from build123d import *

# Parameters (mm, degrees)
F1_DEPTH = 3.175
F2_DEPTH = 4.7498
F3_T     = -1.6002


with BuildPart() as f1:
    # F0 (on Top) → F1 (new body)
    with BuildSketch(Plane.XY):
        with BuildLine():
            Line((-6.9955831819, 8.5962191019), (-38.8090831819, 8.5962191019))
            Line((-38.8090831819, 8.5962191019), (-38.8090831819, 4.6274691019))
            Line((-38.8090831819, 4.6274691019), (-37.2342831819, 4.6274691019))
            ThreePointArc((-37.2342831819, 4.6274691019), (-34.8466831819, 7.0150691019), (-32.4590831819, 4.6274691019))
            Line((-32.4590831819, 4.6274691019), (-29.2840831819, 4.6274691019))
            ThreePointArc((-29.2840831819, 4.6274691019), (-26.8964831819, 7.0150691019), (-24.5088831819, 4.6274691019))
            Line((-24.5088831819, 4.6274691019), (-21.3338831819, 4.6274691019))
            ThreePointArc((-21.3338831819, 4.6274691019), (-18.9462831819, 7.0150691019), (-16.5586831819, 4.6274691019))
            Line((-16.5586831819, 4.6274691019), (-13.3836831819, 4.6274691019))
            ThreePointArc((-13.3836831819, 4.6274691019), (-10.9960831819, 7.0150691019), (-8.6084831819, 4.6274691019))
            Line((-8.6084831819, 4.6274691019), (-6.9955831819, 4.6274691019))
            Line((-6.9955831819, 4.6274691019), (-6.9955831819, 8.5962191019))
        make_face()
        with BuildLine():
            Line((-37.2342831819, 4.6274691019), (-38.8090831819, 4.6274691019))
            Line((-38.8090831819, 4.6274691019), (-38.8090831819, 0.6587191019))
            Line((-38.8090831819, 0.6587191019), (-6.9955831819, 0.6587191019))
            Line((-6.9955831819, 0.6587191019), (-6.9955831819, 4.6274691019))
            Line((-6.9955831819, 4.6274691019), (-8.6084831819, 4.6274691019))
            ThreePointArc((-8.6084831819, 4.6274691019), (-10.9960831819, 2.2398691019), (-13.3836831819, 4.6274691019))
            Line((-13.3836831819, 4.6274691019), (-16.5586831819, 4.6274691019))
            ThreePointArc((-16.5586831819, 4.6274691019), (-18.9462831819, 2.2398691019), (-21.3338831819, 4.6274691019))
            Line((-21.3338831819, 4.6274691019), (-24.5088831819, 4.6274691019))
            ThreePointArc((-24.5088831819, 4.6274691019), (-26.8964831819, 2.2398691019), (-29.2840831819, 4.6274691019))
            Line((-29.2840831819, 4.6274691019), (-32.4590831819, 4.6274691019))
            ThreePointArc((-32.4590831819, 4.6274691019), (-34.8466831819, 2.2398691019), (-37.2342831819, 4.6274691019))
        make_face()
        with BuildLine():
            Line((-37.2342831819, -3.3100308981), (-38.8090831819, -3.3100308981))
            Line((-38.8090831819, -3.3100308981), (-38.8090831819, -7.2787808981))
            Line((-38.8090831819, -7.2787808981), (-6.9955831819, -7.2787808981))
            Line((-6.9955831819, -7.2787808981), (-6.9955831819, -3.3100308981))
            Line((-6.9955831819, -3.3100308981), (-8.6084831819, -3.3100308981))
            ThreePointArc((-8.6084831819, -3.3100308981), (-10.9960831819, -5.6976308981), (-13.3836831819, -3.3100308981))
            Line((-13.3836831819, -3.3100308981), (-16.5586831819, -3.3100308981))
            ThreePointArc((-16.5586831819, -3.3100308981), (-18.9462831819, -5.6976308981), (-21.3338831819, -3.3100308981))
            Line((-21.3338831819, -3.3100308981), (-24.5088831819, -3.3100308981))
            ThreePointArc((-24.5088831819, -3.3100308981), (-26.8964831819, -5.6976308981), (-29.2840831819, -3.3100308981))
            Line((-29.2840831819, -3.3100308981), (-32.4590831819, -3.3100308981))
            ThreePointArc((-32.4590831819, -3.3100308981), (-34.8466831819, -5.6976308981), (-37.2342831819, -3.3100308981))
        make_face()
        with BuildLine():
            Line((-6.9955831819, 0.6587191019), (-38.8090831819, 0.6587191019))
            Line((-38.8090831819, 0.6587191019), (-38.8090831819, -3.3100308981))
            Line((-38.8090831819, -3.3100308981), (-37.2342831819, -3.3100308981))
            ThreePointArc((-37.2342831819, -3.3100308981), (-34.8466831819, -0.9224308981), (-32.4590831819, -3.3100308981))
            Line((-32.4590831819, -3.3100308981), (-29.2840831819, -3.3100308981))
            ThreePointArc((-29.2840831819, -3.3100308981), (-26.8964831819, -0.9224308981), (-24.5088831819, -3.3100308981))
            Line((-24.5088831819, -3.3100308981), (-21.3338831819, -3.3100308981))
            ThreePointArc((-21.3338831819, -3.3100308981), (-18.9462831819, -0.9224308981), (-16.5586831819, -3.3100308981))
            Line((-16.5586831819, -3.3100308981), (-13.3836831819, -3.3100308981))
            ThreePointArc((-13.3836831819, -3.3100308981), (-10.9960831819, -0.9224308981), (-8.6084831819, -3.3100308981))
            Line((-8.6084831819, -3.3100308981), (-6.9955831819, -3.3100308981))
            Line((-6.9955831819, -3.3100308981), (-6.9955831819, 0.6587191019))
        make_face()
    extrude(amount=F1_DEPTH)

    # F0 (on Top) → F2 (join)
    with BuildSketch(Plane.XY):
        with BuildLine():
            Line((-32.4590831819, 4.6274691019), (-37.2342831819, 4.6274691019))
            ThreePointArc((-37.2342831819, 4.6274691019), (-34.8466831819, 2.2398691019), (-32.4590831819, 4.6274691019))
        make_face()
        with BuildLine():
            ThreePointArc((-32.4590831819, 4.6274691019), (-34.8466831819, 7.0150691019), (-37.2342831819, 4.6274691019))
            Line((-37.2342831819, 4.6274691019), (-32.4590831819, 4.6274691019))
        make_face()
        with BuildLine():
            ThreePointArc((-32.4590831819, -3.3100308981), (-34.8466831819, -0.9224308981), (-37.2342831819, -3.3100308981))
            Line((-37.2342831819, -3.3100308981), (-32.4590831819, -3.3100308981))
        make_face()
        with BuildLine():
            Line((-32.4590831819, -3.3100308981), (-37.2342831819, -3.3100308981))
            ThreePointArc((-37.2342831819, -3.3100308981), (-34.8466831819, -5.6976308981), (-32.4590831819, -3.3100308981))
        make_face()
        with BuildLine():
            Line((-24.5088831819, -3.3100308981), (-29.2840831819, -3.3100308981))
            ThreePointArc((-29.2840831819, -3.3100308981), (-26.8964831819, -5.6976308981), (-24.5088831819, -3.3100308981))
        make_face()
        with BuildLine():
            ThreePointArc((-24.5088831819, -3.3100308981), (-26.8964831819, -0.9224308981), (-29.2840831819, -3.3100308981))
            Line((-29.2840831819, -3.3100308981), (-24.5088831819, -3.3100308981))
        make_face()
        with BuildLine():
            Line((-24.5088831819, 4.6274691019), (-29.2840831819, 4.6274691019))
            ThreePointArc((-29.2840831819, 4.6274691019), (-26.8964831819, 2.2398691019), (-24.5088831819, 4.6274691019))
        make_face()
        with BuildLine():
            ThreePointArc((-24.5088831819, 4.6274691019), (-26.8964831819, 7.0150691019), (-29.2840831819, 4.6274691019))
            Line((-29.2840831819, 4.6274691019), (-24.5088831819, 4.6274691019))
        make_face()
        with BuildLine():
            ThreePointArc((-21.3338831819, -3.3100308981), (-18.9462831819, -5.6976308981), (-16.5586831819, -3.3100308981))
            Line((-16.5586831819, -3.3100308981), (-21.3338831819, -3.3100308981))
        make_face()
        with BuildLine():
            Line((-21.3338831819, -3.3100308981), (-16.5586831819, -3.3100308981))
            ThreePointArc((-16.5586831819, -3.3100308981), (-18.9462831819, -0.9224308981), (-21.3338831819, -3.3100308981))
        make_face()
        with BuildLine():
            Line((-21.3338831819, 4.6274691019), (-16.5586831819, 4.6274691019))
            ThreePointArc((-16.5586831819, 4.6274691019), (-18.9462831819, 7.0150691019), (-21.3338831819, 4.6274691019))
        make_face()
        with BuildLine():
            ThreePointArc((-21.3338831819, 4.6274691019), (-18.9462831819, 2.2398691019), (-16.5586831819, 4.6274691019))
            Line((-16.5586831819, 4.6274691019), (-21.3338831819, 4.6274691019))
        make_face()
        with BuildLine():
            Line((-13.3836831819, -3.3100308981), (-8.6084831819, -3.3100308981))
            ThreePointArc((-8.6084831819, -3.3100308981), (-10.9960831819, -0.9224308981), (-13.3836831819, -3.3100308981))
        make_face()
        with BuildLine():
            ThreePointArc((-13.3836831819, -3.3100308981), (-10.9960831819, -5.6976308981), (-8.6084831819, -3.3100308981))
            Line((-8.6084831819, -3.3100308981), (-13.3836831819, -3.3100308981))
        make_face()
        with BuildLine():
            ThreePointArc((-13.3836831819, 4.6274691019), (-10.9960831819, 2.2398691019), (-8.6084831819, 4.6274691019))
            Line((-8.6084831819, 4.6274691019), (-13.3836831819, 4.6274691019))
        make_face()
        with BuildLine():
            Line((-13.3836831819, 4.6274691019), (-8.6084831819, 4.6274691019))
            ThreePointArc((-8.6084831819, 4.6274691019), (-10.9960831819, 7.0150691019), (-13.3836831819, 4.6274691019))
        make_face()
    extrude(amount=F2_DEPTH)

    # F3
    f3_openings = [f1.faces().sort_by_distance(p)[0] for p in [
        (-22.902333, 0.658719, 0),
    ]]
    offset(amount=F3_T, openings=f3_openings, kind=Kind.INTERSECTION)


solid = f1.part
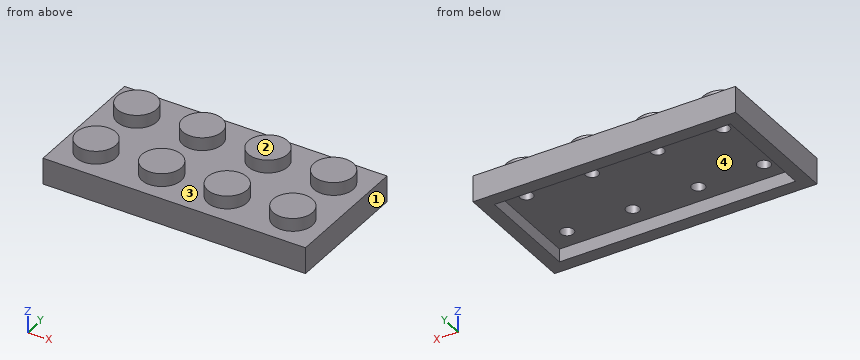
For this review, take the finished solid that the model builds, in its own axes (mm). Face numbers are marked on the shaded views. Coordinates: 2 decimals unless noted, no trailing zeros. Write each loop counter-clockwise with the first axis right and the second up, starting at its lowest first coordinate (ties: lowest second). Pieces come first, ordered by that corner, then holes. Notation, with made-up numbers: (-25, 83) -> (21, 83) arc R9 cw to (21, 96) -> close; hole circle Ø1 at (46.5, 49.5). An arc over 180 degrees is marked (long way). Write each question's results on one line, items separated by ' | '. Start each with the question number.
1) Wall thickness on L1, parallel to X at y = -3.25, z = 4.25; L2, parallel to X at y = 5.25, z = 4.1; L3, parallel to X at y = -3.75, z = 3.05: over which ranges is each line inside the solid? List them lowest first. Write a range as [from, to].
2) Consider section D-D (z = 3.95). Write out the cut boundary in (x, y).
3) Consider section C-C (y = -0.5). Write out the cut boundary in (x, z) (3 decimals).
4) Consider section B-B (x = -11). Write out the cut boundary in (y, z) (3 decimals).
5) The part is to be moulded in two halves that separate along X. For the marked faces 1, 2, 3 and 4, say which applies: +X half, -X half, draft (parallel to the pull), parting line (faces both ways), or undercut.
6) Insertion check: pin 1 (1.7 mm diameter, centred on x = -35, y = 5, fed in from -Z); pin 2 (1.3 mm diameter, centred on x = -34.85, y = -3.31, fed in from -Z). Each pin has a flat end and moves straight along its axis. Give the tip position at first contact, or say it passes through.
7) Consider section A-A (z = 0.7). Write out the cut boundary in (x, y), plus the area to 3 significant figures.
Geometry says:
1) L1: [-37.23, -32.46], [-29.28, -24.51], [-21.33, -16.56], [-13.38, -8.61] | L2: [-37.15, -32.54], [-29.2, -24.59], [-21.25, -16.64], [-13.3, -8.69] | L3: [-38.81, -35.5], [-34.19, -27.55], [-26.24, -19.6], [-18.29, -11.65], [-10.34, -7]
2) outline: circle Ø4.78 at (-34.85, -3.31); circle Ø4.78 at (-34.85, 4.63); circle Ø4.78 at (-26.9, -3.31); circle Ø4.78 at (-26.9, 4.63); circle Ø4.78 at (-18.95, -3.31); circle Ø4.78 at (-18.95, 4.63); circle Ø4.78 at (-11, -3.31); circle Ø4.78 at (-11, 4.63)
3) outline: (-38.809, 0) -> (-37.209, 0) -> (-37.209, 1.575) -> (-8.596, 1.575) -> (-8.596, 0) -> (-6.996, 0) -> (-6.996, 3.175) -> (-38.809, 3.175) -> close
4) outline: (-7.279, 0) -> (-5.679, 0) -> (-5.679, 1.575) -> (-4.097, 1.575) -> (-4.097, 3.15) -> (-2.523, 3.15) -> (-2.523, 1.575) -> (3.84, 1.575) -> (3.84, 3.15) -> (5.415, 3.15) -> (5.415, 1.575) -> (6.996, 1.575) -> (6.996, 0) -> (8.596, 0) -> (8.596, 3.175) -> (7.015, 3.175) -> (7.015, 4.75) -> (2.24, 4.75) -> (2.24, 3.175) -> (-0.922, 3.175) -> (-0.922, 4.75) -> (-5.698, 4.75) -> (-5.698, 3.175) -> (-7.279, 3.175) -> close
5) face 1: +X half | face 2: draft | face 3: undercut | face 4: undercut
6) pin 1: z = 1.57 | pin 2: z = 3.15
7) outline: (-38.81, -7.28) -> (-7, -7.28) -> (-7, 8.6) -> (-38.81, 8.6) -> close; hole (-37.21, -5.68) -> (-8.6, -5.68) -> (-8.6, 7) -> (-37.21, 7) -> close | area: 142 mm^2
